Job drawing, mm, ordinate dimensions from the low corner. One solid piece. Give positions to 0.01 mm unless a question says otherwise; leave off trailing zeros. Loops run counter-clockwise (first coordinate to the right, second up) from the corner with the lowest first, then second, coordinate; pieces in that order, holes last.
Item 1: Probe probe 1 along X at (y, z) = (3.8, 9.5) (1 decimal); probe 2 along Z at (x, y) = (25, 4.15) (1 decimal); probe 3 along Z at (x, y) = (28, 0.8) (1 decimal). List the from-to ranges inside material, lowest first.
Item 2: Drop flat-ended pins along their axis: P1, Ø1.5, axis at y = 1.5, z = 45.5, coming from the -X side; P2, Ø5, axis at x = 4.89, z = 61.43, coming from the +Y side; P3, Ø1.5, axis at x = 6, z = 45.5, coming from the +Y side; P4, Ø3, axis at x = 24.5, y = 1.5, coming from the +Z side (1 decimal). Give the stop position or say it passes through.
Item 3: Saw through at C-C on y = 1.2. Give the number of separate pieces and of enclosed holes in the cut face, plus the area to 3 significant figures.
Item 4: Saw through at D-D on x = 19.5. Give the cut face in (y, z).
Item 5: Saw through at A-A on x = 4. Give the cut face in (y, z).
Item 6: Saw through at B-B on x = 28.5. Give the cut face in (y, z).
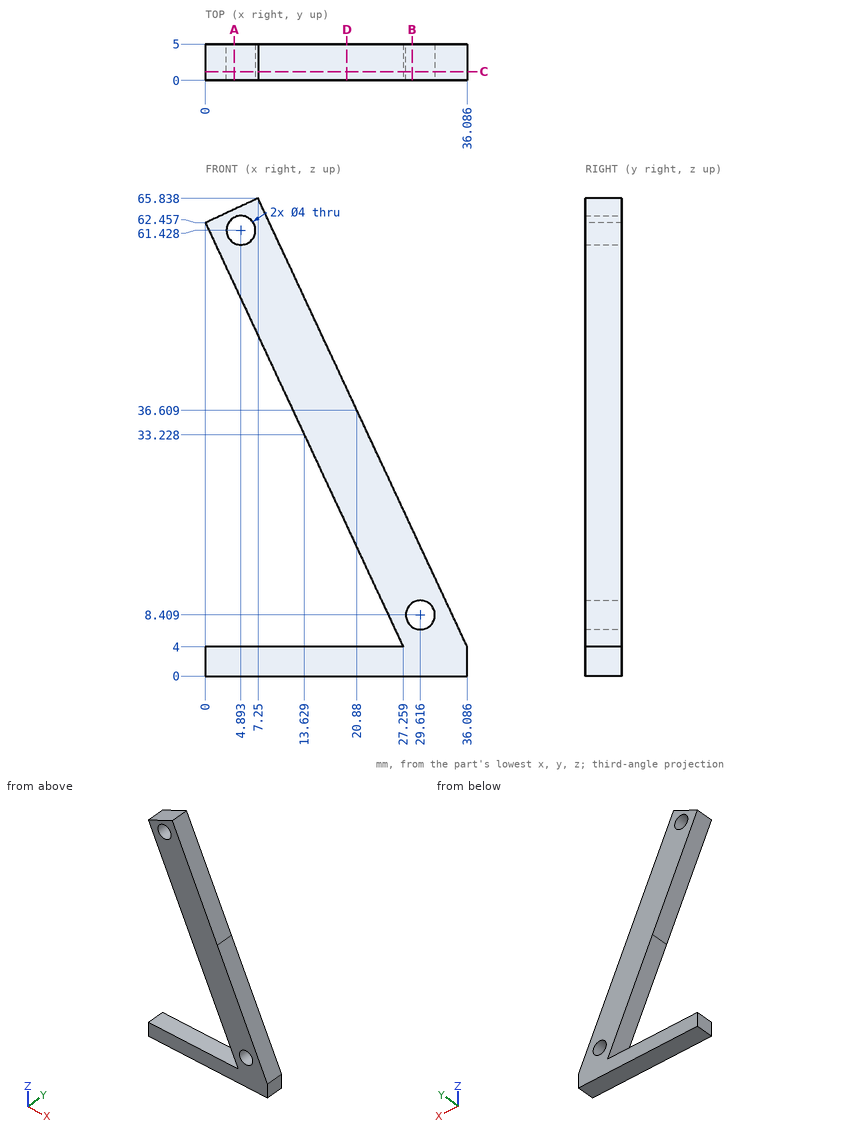
Results below:
1. probe 1: x = 24.7 to 27.9, 31.3 to 33.5
1. probe 2: z = 0 to 4, 8.8 to 27.8
1. probe 3: z = 0 to 7.2, 9.6 to 21.3
2. P1: stops at x = 7.56
2. P2: stops at y = 5
2. P3: passes through
2. P4: stops at z = 32.1
3. separate pieces: 1
3. enclosed holes: 2
3. area: 650 mm2
4. outline: (0, 0) - (5, 0) - (5, 4) - (0, 4) - close; (0, 20.64) - (5, 20.64) - (5, 39.57) - (0, 39.57) - close
5. outline: (0, 0) - (5, 0) - (5, 4) - (0, 4) - close; (0, 53.88) - (5, 53.88) - (5, 59.64) - (0, 59.64) - close; (0, 63.22) - (5, 63.22) - (5, 64.32) - (0, 64.32) - close
6. outline: (0, 0) - (5, 0) - (5, 6.75) - (0, 6.75) - close; (0, 10.07) - (5, 10.07) - (5, 20.27) - (0, 20.27) - close
